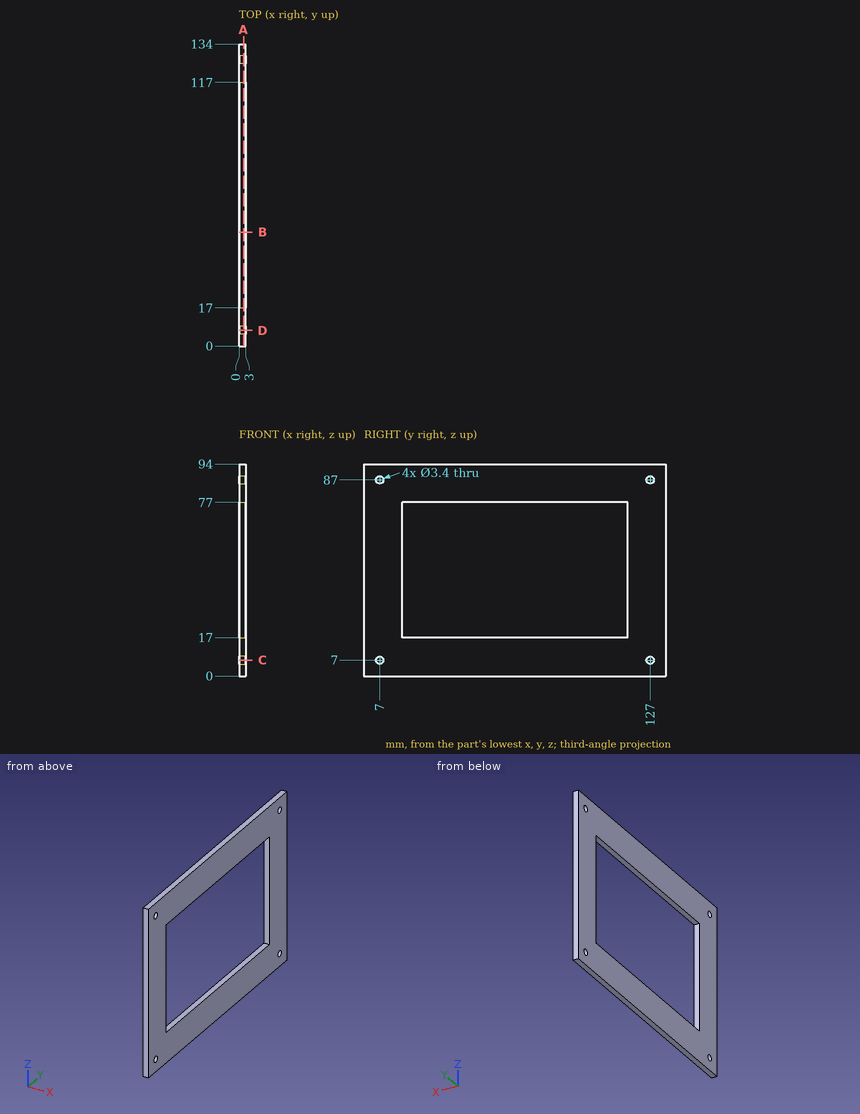
Drawing for the job (mm, zero at the part's lowest x, y, z). Round coordinates to 2 decimals unless told otherwise and drop trailing zeros. Write each loop counter-clockwise with the first axis right and the second up, starting at its lowest first coordinate (ties: lowest second). Pieces come first, ordered by that corner, then holes. Notation, with made-up numbers: M -2,-18.5 L 4,-18.5 A28 cw 4,20.5 Z; hole C 25.5,-24 d11. An arc over 180 degrees is marked long. Answer in a Markdown table with one row per item.
1. Saw through at D-D (y = 7). List the corners of the cut face in (x, z), and give its area (3 significant figures).
Geometry check:
| item | result |
|---|---|
| outline | M 0,0 L 3,0 L 3,5.3 L 0,5.3 Z; M 0,8.7 L 3,8.7 L 3,85.3 L 0,85.3 Z; M 0,88.7 L 3,88.7 L 3,94 L 0,94 Z |
| area | 262 mm2 |
2. Saw through at C-C (z = 7). List the corners of the cut face in (x, y).
Geometry check:
| item | result |
|---|---|
| outline | M 0,0 L 3,0 L 3,5.3 L 0,5.3 Z; M 0,8.7 L 3,8.7 L 3,125.3 L 0,125.3 Z; M 0,128.7 L 3,128.7 L 3,134 L 0,134 Z |
3. Flat gauge pin, fed straight in: P1, Ø4, axis at y = 7, z = 87, coming from the +X side. Where does the tip first touch, or does it go through?
Geometry check:
| item | result |
|---|---|
| P1 | x = 3 |
4. Probe L1, parallel to Y at x = 1.05, z = 7; L2, parallel to Z at x = 2.1, y = 127; L3, parallel to Z at x = 1.55, y = 56.5. List the from-to ranges inside material, lowest first. Write a range as [from, to].
Geometry check:
| item | result |
|---|---|
| L1 | [0, 5.3], [8.7, 125.3], [128.7, 134] |
| L2 | [0, 5.3], [8.7, 85.3], [88.7, 94] |
| L3 | [0, 17], [77, 94] |
5. Saw through at B-B (y = 50.5). List the corners of the cut face in (x, z).
Geometry check:
| item | result |
|---|---|
| outline | M 0,0 L 3,0 L 3,17 L 0,17 Z; M 0,77 L 3,77 L 3,94 L 0,94 Z |
6. Saw through at A-A (x = 2.05). List the corners of the cut face in (y, z).
Geometry check:
| item | result |
|---|---|
| outline | M 0,0 L 134,0 L 134,94 L 0,94 Z; hole C 7,7 d3.4; hole C 7,87 d3.4; hole M 17,17 L 117,17 L 117,77 L 17,77 Z; hole C 127,7 d3.4; hole C 127,87 d3.4 |
